```python
from build123d import *

# Parameters (mm, degrees)
SKETCH2_W = 2.05
SKETCH2_H = 1


with BuildPart() as part:
    # Sketch1 → Revolve1 (revolve)
    with BuildSketch(Plane(origin=(0, 0, 0), x_dir=(0, 0, -1), z_dir=(1, 0, 0))):
        Polygon((4.65, 1), (4.65, 4.3), (4.5, 4.3), (4.5, 12.5), (5.4, 12.5), (5.4, 6.2), (5.6, 6.2), (5.6, 0), (4.8, 0), align=None)
    revolve(axis=Axis((0, 0, 0), (0, 1, 0)))

    # Sketch2 → Revolve2 (revolve)
    with BuildSketch(Plane(origin=(0, 0, 0), x_dir=(0, 0, -1), z_dir=(1, 0, 0))):
        with Locations((6.625, 5.7)):
            Rectangle(SKETCH2_W, SKETCH2_H)
    revolve(axis=Axis((0, 0, 0), (0, 1, 0)))

    # Sketch3 → Revolve-Thin1 (revolve)
    with BuildSketch(Plane(origin=(0, 0, 0), x_dir=(0, 0, -1), z_dir=(1, 0, 0))):
        Polygon((7.9, 10.3), (7.9, 9.3), (7.65, 8), (7.65, 5.2), (8.25, 1.5), (8.25, 0), (9.25, 0), (9.25, 1.580554938), (8.65, 5.280554938), (8.65, 7.904719082), (8.9, 9.204719082), (8.9, 10.3), align=None)
    revolve(axis=Axis((0, 0, 0), (0, 1, 0)))


solid = part.part
```
Part model, mm, in its own coordinate system. A direction names the side the tool comes from. Round coordinates to 2 decimals unless told otherwise and drop trailing zeros. Order: outer loops, then holes, each group sorted by start corner. A loop starts at its lowest first (then second) coordinate and runs counter-clockwise, first axis right, second up. Notation, with made-up numbers: M -8.5,62.25 L 12.5,62.25 A14 cw 12.5,76.25 Z; hole C 39.5,40.25 d8. An arc over 180 degrees is marked long. Put each result on its own line as item: value. Start each with the question number.
1. Tool access for faces 1 (the face through (-2.6, 6.61, -8.25)), 2 (the face through (5.27, 9.31, 1.17)), 3 (the face through (-3.92, 2.67, -2.5)), 4 (the face through (-3, 0, -4)), 5 (the face through (-4, 12.5, -3)): list every direction of +Z, -Z, +X, -X, +Y, -Y with a clear straight run to the whole face (end or side of a thin tool).
2. Drop flat-ended pins along their axis: pin 1 (5 mm diameter, centred on x = -3.5, y = 7, fed in from +Z); pin 2 (1 mm diameter, centred on x = 4, z = 0.5, fed in from -Y); pin 3 (6 mm diameter, centred on y = 9, z = 1.5, fed in from +X). Give the stop position or say it passes through.
3. Slice it at A-A on y = 10. List the corners of the cut face in (x, z), then the cut area to 3 significant figures.
4. Slice it at C-C on y = 1.25. List the corners of the cut face in (x, z).
5. Slice it at B-B on y = 11.5. List the corners of the cut face in (x, z).
6. Drill centre lines: probe 1 along Z at (x, y) = (0, 7.25); probe 2 along Z at (x, y) = (0, 9.6); probe 3 along X at (y, z) = (5, 3.5). Where is each one in solid material? Low to high. Write a range as [from, to].
7. Two-plate mould, pull along Z, no slides. Class faces 6 (the face through (-8.67, 4.69, 1.14)), 7 (the face through (8, 10.3, 1)), 8 (the face through (3.16, 0.74, -7.62)): +Z half, -Z half, draft (parallel to the pull), parting line (faces both ways), or undercut.
Findings:
1. face 1: none
1. face 2: +Y
1. face 3: -Y
1. face 4: +Z, -Z, +X, -X, -Y
1. face 5: +Z, -Z, +X, -X, +Y
2. pin 1: z = 8.64
2. pin 2: y = 4.3
2. pin 3: x = 8.9
3. outline: C 0,0 d17.8; C 0,0 d10.8; hole C 0,0 d15.8; hole C 0,0 d9
3. area: 80.8 mm2
4. outline: C 0,0 d18.5; C 0,0 d11.2; hole C 0,0 d16.5; hole C 0,0 d9.3
5. outline: C 0,0 d10.8; hole C 0,0 d9
6. probe 1: [-8.65, -7.65], [-5.4, -4.5], [4.5, 5.4], [7.65, 8.65]
6. probe 2: [-8.9, -7.9], [-5.4, -4.5], [4.5, 5.4], [7.9, 8.9]
6. probe 3: [-7.96, -6.84], [-4.37, -2.83], [2.83, 4.37], [6.84, 7.96]
7. face 6: parting line
7. face 7: draft
7. face 8: undercut
